Design review of the part built by this model. Coordinates are the model's own, in mm. Give positions to 0.01 mm unless a question says otherwise; leave off trailing zeros. Use a Markdown table: item, result. Add a question column.
```python
from build123d import *

# Parameters (mm, degrees)
SWEEP1_PROFILE_R     = 13.49375
CUT_SWEEP1_PROFILE_R = 9.525


with BuildPart() as part:
    # Sweep1: sweep along a curve in space
    with BuildLine() as sweep1_path:
        Line((23.5, 73, -27), (23.5, 73, 0))
        ThreePointArc((23.5, 73, 0), (74.341792088, 92.360177629, 104.205083686), (183.308831735, 133.854018751, 119.133217723))
        ThreePointArc((313.846862771, 135.151241794, 107.30619915), (247.643313282, 145.663188238, 104.129125644), (183.308831735, 133.854018751, 119.133217723))
        Line((323.696537416, 131.80975388, 109.239001446), (313.846862771, 135.151241794, 107.30619915))
        Line((323.696537416, 131.80975388, 109.239001446), (342.615480312, 125.391529797, 112.951466843))
    # Sweep1 profile (on start of the path) → Sweep1 (sweep)
    with BuildSketch(Plane(origin=(23.5, 73, -27), x_dir=(1, 0, 0), z_dir=(0, 0, 1))):
        Circle(SWEEP1_PROFILE_R)
    sweep(path=sweep1_path.line)

    # Cut-Sweep1: sweep along a curve in space
    with BuildLine() as cut_sweep1_path:
        Line((23.5, 73, -27), (23.5, 73, 0))
        ThreePointArc((23.5, 73, 0), (74.341792088, 92.360177629, 104.205083686), (183.308831735, 133.854018751, 119.133217723))
        ThreePointArc((313.846862771, 135.151241794, 107.30619915), (247.643313282, 145.663188238, 104.129125644), (183.308831735, 133.854018751, 119.133217723))
        Line((323.696537416, 131.80975388, 109.239001446), (313.846862771, 135.151241794, 107.30619915))
        Line((323.696537416, 131.80975388, 109.239001446), (342.615480312, 125.391529797, 112.951466843))
    # Cut-Sweep1 profile (on start of the path) → Cut-Sweep1 (sweep, cut)
    with BuildSketch(Plane(origin=(23.5, 73, -27), x_dir=(1, 0, 0), z_dir=(0, 0, 1))):
        Circle(CUT_SWEEP1_PROFILE_R)
    sweep(path=cut_sweep1_path.line, mode=Mode.SUBTRACT)


solid = part.part
```
(1) Insertion check: pin 1 (11.5 mm diameter, centred on x = 23.5, y = 73, fed in from +Z); pin 2 (4 mm diameter, centred on x = 91, y = 112.5, fed in from -Z); pin 3 (4 mm diameter, centred on x = 222.5, y = 133, fed in from +Z). Each pin has a flat end and moves straight along its axis. Give the tip position at first contact, or say it passes through.
(2) For line 1 along Y through (x, z) = (23.5, -9.75) (3 decimals); line 2 along Z through (x, y) = (126.5, 113); line 3 along X through (y, z) = (79, 32.5), list the stretches that pass through material, from the lowest coordinate up.
(3) Mouldability with a two-part tool opening along X and no side actions: class faces 1 (the face through (28.62, 81.03, -13.31)), 2 (the face through (21.74, 86.38, -13.31)), 3 (the face through (14, 70, -27)) as +X half, -X half, draft (parallel to the pull), parting line (faces both ways), or undercut.
Answers follow:
| question | item | result |
|---|---|---|
| 1 | pin 1 | z = 70.97 |
| 1 | pin 2 | z = 107.95 |
| 1 | pin 3 | z = 118.65 |
| 2 | line 1 | 59.506 to 63.475, 82.525 to 86.494 |
| 2 | line 2 | 112.32 to 116.34, 135.5 to 139.5 |
| 2 | line 3 | 14.47 to 18.9, 36.25 to 40.73 |
| 3 | face 1 | undercut |
| 3 | face 2 | parting line |
| 3 | face 3 | draft |
